from build123d import *

# Parameters (mm, degrees)
SKETCH1_R               = 2
BOSS_EXTRUDE1_DEPTH     = 9
BOSS_EXTRUDE2_DEPTH     = 40.25
CUT_EXTRUDE1_DEPTH      = 50
SKETCH6_W               = 3.25
SKETCH6_H               = 24.113806611
CUT_EXTRUDE2_DEPTH      = 10.6
SKETCH7_R               = 1.8
CUT_EXTRUDE3_DEPTH      = 39.5
CUT_EXTRUDE3_DEPTH_BACK = 39.5
CUT_EXTRUDE4_DEPTH      = 20.85
SKETCH9_R               = 4.05
CUT_EXTRUDE5_DEPTH      = 2.4
CUT_EXTRUDE6_DEPTH      = 6.5


with BuildPart() as part:
    # Sketch1 → Boss-Extrude1 (new body)
    with BuildSketch(Plane.XY):
        with BuildLine():
            Line((0, 0), (-7.3836, 0))
            Line((-7.3836, 0), (-26.6, 47.5))
            Line((-26.6, 47.5), (-26.6, 54.25))
            ThreePointArc((-26.6, 54.25), (-34.1, 61.75), (-41.6, 54.25))
            Line((-41.6, 54.25), (-41.6, 51.364872675))
            ThreePointArc((-41.6, 51.364872675), (-42.771572875, 48.53644555), (-45.6, 47.364872675))
            Line((-45.6, 47.364872675), (-60.316706428, 47.364872675))
            ThreePointArc((-60.316706428, 47.364872675), (-65.973560677, 49.708018426), (-68.316706428, 55.364872675))
            Line((-68.316706428, 55.364872675), (-68.316706428, 78.864872675))
            ThreePointArc((-68.316706428, 78.864872675), (-65.973560677, 84.521726925), (-60.316706428, 86.864872675))
            Line((-60.316706428, 86.864872675), (-48.816706428, 86.864872675))
            ThreePointArc((-48.816706428, 86.864872675), (-34.212822301, 98.749840665), (-19.5, 87))
            Line((-19.5, 87), (-8, 87))
            ThreePointArc((-8, 87), (-2.343145751, 84.656854249), (0, 79))
            Line((0, 79), (0, 0))
        make_face()
        with Locations((-50.316706428, 78.114872675)):
            Circle(SKETCH1_R, mode=Mode.SUBTRACT)
        with Locations((-18.316706428, 78.114872675)):
            Circle(SKETCH1_R, mode=Mode.SUBTRACT)
        with Locations((-50.316706428, 53.614872675)):
            Circle(SKETCH1_R, mode=Mode.SUBTRACT)
        with Locations((-18.316706428, 53.614872675)):
            Circle(SKETCH1_R, mode=Mode.SUBTRACT)
    extrude(amount=BOSS_EXTRUDE1_DEPTH)

    # Sketch3 → Boss-Extrude2 (add)
    with BuildSketch(Plane(origin=(0, 0, 0), x_dir=(-1, 0, 0), z_dir=(0, 0, -1))):
        with BuildLine():
            Line((0, 0), (5.4, 0))
            Line((5.4, 0), (5.4, 58.675))
            ThreePointArc((5.4, 58.675), (6.886433085, 62.263566915), (10.475, 63.75))
            Line((10.475, 63.75), (57.6, 63.75))
            Line((57.6, 63.75), (57.6, 69.45))
            ThreePointArc((57.6, 69.45), (34.1, 77.587816557), (10.6, 69.45))
            Line((10.6, 69.45), (10.6, 69.1))
            Line((10.6, 69.1), (10.375, 69.1))
            ThreePointArc((10.375, 69.1), (3.038767145, 66.061232855), (0, 58.725))
            Line((0, 58.725), (0, 0))
        make_face()
    extrude(amount=BOSS_EXTRUDE2_DEPTH)

    # Sketch5 → Cut-Extrude1 (cut)
    with BuildSketch(Plane.XY.offset(9)):
        with BuildLine():
            Line((-28.716706428, 84.614872675), (-28.716706428, 81.614872675))
            ThreePointArc((-28.716706428, 81.614872675), (-34.216706428, 76.114872675), (-39.716706428, 81.614872675))
            Line((-39.716706428, 81.614872675), (-39.716706428, 84.614872675))
            ThreePointArc((-39.716706428, 84.614872675), (-34.216706428, 90.114872675), (-28.716706428, 84.614872675))
        make_face()
    extrude(amount=-CUT_EXTRUDE1_DEPTH, mode=Mode.SUBTRACT)

    # Sketch6 → Cut-Extrude2 (cut)
    with BuildSketch(Plane(origin=(0, 0, 0), x_dir=(0, 0, -1), z_dir=(1, 0, 0))):
        with BuildLine():
            Line((37, 58.725), (37, 36.056406461))
            ThreePointArc((37, 36.056406461), (32.178877657, 28.715102977), (23.526315789, 30.222130056))
            ThreePointArc((23.526315789, 30.222130056), (7.877678535, 29.618078863), (8.691491696, 13.978947368))
            ThreePointArc((8.691491696, 13.978947368), (10.853899034, 5.156725387), (3.37621293, 0))
            Line((3.37621293, 0), (37.9285464, 0))
            Line((37.9285464, 0), (40.25, 0))
            Line((40.25, 0), (40.25, 58.725))
            Line((40.25, 58.725), (37, 58.725))
        make_face()
        with BuildLine():
            Line((3.096104185, 37.603623706), (0.26725, 40.431623706))
            ThreePointArc((0.26725, 40.431623706), (-2.207623706, 40.43125), (-2.20725, 37.956376294))
            Line((-2.20725, 37.956376294), (0.621604185, 35.128376294))
            ThreePointArc((0.621604185, 35.128376294), (3.096477891, 35.12875), (3.096104185, 37.603623706))
        make_face()
        with BuildLine():
            ThreePointArc((31.73275, 40.431623706), (34.207623706, 40.43125), (34.20725, 37.956376294))
            Line((34.20725, 37.956376294), (31.378395815, 35.128376294))
            ThreePointArc((31.378395815, 35.128376294), (28.903522109, 35.12875), (28.903895815, 37.603623706))
            Line((28.903895815, 37.603623706), (31.73275, 40.431623706))
        make_face()
        with BuildLine():
            ThreePointArc((0.26725, 3.968376294), (-2.207623706, 3.96875), (-2.20725, 6.443623706))
            Line((-2.20725, 6.443623706), (0.621604185, 9.271623706))
            ThreePointArc((0.621604185, 9.271623706), (3.096477891, 9.27125), (3.096104185, 6.796376294))
            Line((3.096104185, 6.796376294), (0.26725, 3.968376294))
        make_face()
        with Locations((38.625, 70.781903306)):
            Rectangle(SKETCH6_W, SKETCH6_H)
    extrude(amount=-CUT_EXTRUDE2_DEPTH, mode=Mode.SUBTRACT)

    # Sketch7 → Cut-Extrude3 (cut, two sides)
    with BuildSketch(Plane(origin=(0, 86.864872675, 0), x_dir=(1, 0, 0), z_dir=(0, 1, 0))) as cut_extrude3_sk:
        with Locations((-51.6, 34.75)):
            Circle(SKETCH7_R)
        with Locations((-51.6, 6)):
            Circle(SKETCH7_R)
        with Locations((-16.745188355, 6.033054654)):
            Circle(SKETCH7_R)
        with Locations((-16.799718585, 34.78300294)):
            Circle(SKETCH7_R)
        Polygon((-13.833, -9), (-11.1, -5.12), (-7.3, -5.12), (-4.5, -9), align=None)
        Polygon((-63.816706428, -9), (-61.016706428, -5.217), (-57.216706428, -5.217), (-54.486706428, -9), align=None)
    extrude(amount=CUT_EXTRUDE3_DEPTH, mode=Mode.SUBTRACT)
    extrude(cut_extrude3_sk.sketch, amount=-CUT_EXTRUDE3_DEPTH_BACK, mode=Mode.SUBTRACT)

    # Sketch8 → Cut-Extrude4 (cut)
    with BuildSketch(Plane(origin=(0, 86.864872675, 0), x_dir=(1, 0, 0), z_dir=(0, 1, 0))):
        Polygon((-48.135898385, 34.75), (-49.867949192, 37.75), (-53.332050808, 37.75), (-55.064101615, 34.75), (-53.332050808, 31.75), (-49.867949192, 31.75), align=None)
        Polygon((-48.135898385, 6), (-49.867949192, 9), (-53.332050808, 9), (-55.064101615, 6), (-53.332050808, 3), (-49.867949192, 3), align=None)
        Polygon((-18.469686835, 9.036434754), (-15.005594549, 9.044474276), (-13.266585975, 6.048502117), (-14.991669687, 3.044490435), (-18.455761973, 3.036450912), (-20.194770547, 6.032423072), align=None)
        Polygon((-18.522485268, 31.786373486), (-20.261493842, 34.782345646), (-18.53641013, 37.786357328), (-15.072317844, 37.79439685), (-13.33330927, 34.798424691), (-15.058392982, 31.794413009), align=None)
    extrude(amount=-CUT_EXTRUDE4_DEPTH, mode=Mode.SUBTRACT)

    # Sketch9 → Cut-Extrude5 (cut)
    with BuildSketch(Plane(origin=(0, 0, 0), x_dir=(-1, 0, 0), z_dir=(0, 0, -1))):
        with Locations((18.316706428, 78.114872675)):
            Circle(SKETCH9_R)
        with Locations((50.316706428, 78.114872675)):
            Circle(SKETCH9_R)
        with Locations((18.316706428, 53.614872675)):
            Circle(SKETCH9_R)
        with Locations((50.316706428, 53.614872675)):
            Circle(SKETCH9_R)
    extrude(amount=-CUT_EXTRUDE5_DEPTH, mode=Mode.SUBTRACT)

    # Sketch10 → Cut-Extrude6 (cut)
    with BuildSketch(Plane(origin=(0, 0, 0), x_dir=(-1, 0, 0), z_dir=(0, 0, -1))):
        Polygon((26.6, 47.5), (5.4, 47.5), (5.4, 0), (7.3836, 0), align=None)
    extrude(amount=-CUT_EXTRUDE6_DEPTH, mode=Mode.SUBTRACT)


solid = part.part
Verification items for the finished model (mm, model axes). A direction names the side the tool comes from. Round coordinates to 2 decimals unless told otherwise and drop trailing zeros. Loops run counter-clockwise (first coordinate to the right, second up) from the corner with the lowest first, then second, coordinate; pieces in that order, holes last. Notation, with made-up numbers: (14.5, -8.75) - (34.5, -8.75) arc R12 cw to (34.5, 5.25) - close; hole circle Ø6 at (-1, -33.5). An arc over 180 degrees is marked (long way). Write item = value, one per line.
Q1. Depth check by flat-ended pin: pin 1 (10 mm diameter, centred on x = -12, z = -30, fed in from -Y); pin 2 (2 mm diameter, centred on y = 80, z = -13.5, fed in from -X); pin 3 (6.5 mm diameter, centred on x = -50.32, y = 53.61, fed in from -Z); pin 4 (6.5 mm diameter, centred on y = 65.5, z = -13.5, fed in from +X). Enter the tip coordinate at first touch or a pass-through.
Here are the results:
pin_1 = 62.37
pin_2 = through
pin_3 = 2.4
pin_4 = -0.62
Q2. Sectioned sample at A-A on x = -34.1. Record the boundary of the cut face in (y, z), plus the area to 3 significant figures.
Here are the results:
outline = (61.75, 0) - (63.75, 0) - (63.75, -40.25) - (76.12, -40.25) - (76.12, 9) - (61.75, 9) - close; (90.11, 0) - (98.75, 0) - (98.75, 9) - (90.11, 9) - close
area = 705 mm^2
Q3. Material ranges on L1, parallel to Z at x = -51.6, y = 64.65; L2, parallel to Z at x = -54, y = 66.5; L3, parallel to X at y = 80, z = 1.5, recorded low to high.
Here are the results:
L1 = -40.25 to -36.55, -32.95 to -7.8, -4.2 to 9
L2 = -40.25 to -36.59, -32.91 to -7.84, -4.16 to 9
L3 = -68.24 to -53.9, -46.73 to -39.47, -28.96 to -21.9, -14.73 to -0.06
Q4. Sectioned sample at B-B on y = 23. Record the boundary of the cut face in (x, z).
Here are the results:
outline = (-16.69, 6.5) - (-5.4, 6.5) - (-5.4, -5.03) - (0, -5.03) - (0, 9) - (-16.69, 9) - close
Q5. Tool access check on faces 5 (the flat face through (-16, 53, 2.4)), 6 (the flat face through (-55.87, 67.39, 7.08)), 7 (the flat face through (-26.6, 51, 4)), 8 (the flat face through (-54.186, 69.233, -36.271)). Record the directions out of +Z, -Z, +X, -X, +Y, -Y that give a thin tool (end or side, any length) a straight path to the whole face; none if there is none.
Here are the results:
face_5 = -Z
face_6 = +Z, +Y, -Y
face_7 = +Z, -Z, -Y
face_8 = +Y
Q6. Mould release check, pull along X, two halves, no side actions. Record for faces 1 (the flat face through (-48.99, 70.52, -36.23)), 2 (the flat face through (-53, 86.865, 3)), 3 (the flat face through (-57.6, 67, -20)), 4 (the cylindrical face through (-47.33, 56.35, 1.18)): +X half, -X half, draft (parallel to the pull), parting line (faces both ways), or undercut.
Here are the results:
face_1 = undercut
face_2 = draft
face_3 = -X half
face_4 = undercut
